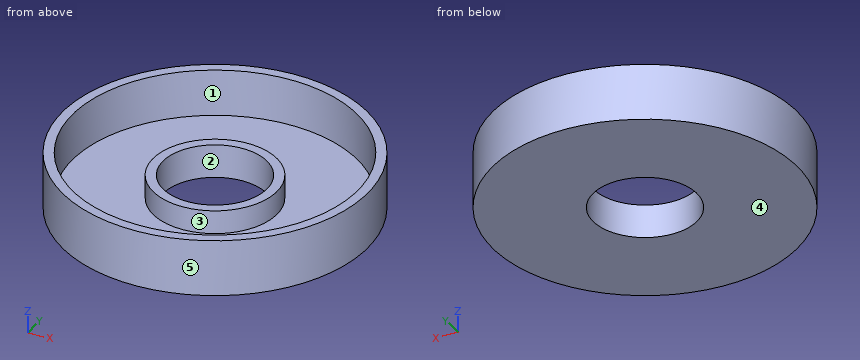
Autodesk Inventor part; units mm, degrees
ref_plane "YZ Plane" through (0, 0, 0) normal (1, 0, 0) x (0, 1, 0)
ref_plane "XZ Plane" through (0, 0, 0) normal (0, 1, 0) x (-1, 0, 0)
ref_plane "XY Plane" through (0, 0, 0) normal (0, 0, 1) x (1, 0, 0)
sketch "Sketch1" plane through (0, 0, 0) normal (0, 0, 1) x (1, 0, 0)
  circle A0 centre (0, 0) radius 61.5
  dimension "d0" = 123
extrude "Extrusion1" add sketch "Sketch1" along normal blind 4
sketch "Sketch2" plane through (0, 0, 4) normal (0, 0, 1) x (1, 0, 0)
  circle A0 centre (0, 0) radius 61.5
  circle A1 centre (0, 0) radius 57.5
  dimension "d12" = 115
extrude "Extrusion2" add sketch "Sketch2" along normal blind 18.85
sketch "Sketch3" plane through (0, 0, 0) normal (0, 0, -1) x (-1, 0, 0)
  circle A0 centre (0, 0) radius 21
  dimension "d6" = 42
extrude "Extrusion3" cut sketch "Sketch3" against normal through all
sketch "Sketch4" plane through (0, 0, 4) normal (0, 0, 1) x (1, 0, 0)
  circle A0 centre (0, 0) radius 21
  circle A1 centre (0, 0) radius 25
  dimension "d9" = 4
extrude "Extrusion4" add sketch "Sketch4" along normal blind 9.5
properties part number "stator_housing"
The listing builds one solid part. Answer for the finished solid, in the listing's coordinates (mm). Face numbers are marked on the shaded views. A direction names the side the tool comes from. Coordinates: 2 decimals unless noted, no trailing zeros. Order: outer loops, then holes, each group sorted by start corner. A loop starts at its lowest first (then second) coordinate and runs counter-clockwise, first axis right, second up.
Q1. Consider line 1 (Y direction, x = 0, z = 6.75); line 2 (Z direction, x = 29, y = -17.5); line 3 (Y direction, x = 0, z = 3.25). Determine where each line is inside the solid, lowest interval first.
Q2. Given P1, Ø15, axis at x = 12, y = -7, coming from the +Z side; P2, Ø12, axis at x = 11.5, z = 13.5, coming from the +Y side; P3, Ø10, axis at x = -47.5, z = 6.5, coming from the -Y side; P4, Ø5, axis at x = 44, y = -33, coming from the -Z side, each flat-ended and moving along its own axis, determine where each tip first touches the part or whether it passes through.
Q3. A cutting plane is placed at C-C, the plane z = 12. Write down the section's boundary in (x, y), and give its area (3 significant figures).
Q4. A cutting plane is placed at A-A, the plane x = 0. Write down the section's boundary in (y, z), and give its area (3 significant figures).
Q5. For a pull along Y with two mould halves and no side action, classify the marked faces 3, 4 and 5 as pulls with the +Y half, pulls with the -Y half, needs draft (parallel to the pull), parting line crosses it, or undercut.
Q6. Which of the six approach directions +Z, -Z, +X, -X, +Y, -Y give full straight-line access (tool end or side, diameter ignored) to the marked faces 1 and 2?
Q7. A cutting plane is placed at D-D, the plane x = 43.5. Write down the section's boundary in (y, z), and give its area (3 significant figures).
Answers follow:
1. line 1: y = -61.5 to -57.5, -25 to -21, 21 to 25, 57.5 to 61.5
1. line 2: z = 0 to 4
1. line 3: y = -61.5 to -21, 21 to 61.5
2. P1: stops at z = 13.5
2. P2: stops at y = 61.25
2. P3: stops at y = -44.45
2. P4: stops at z = 0
3. outline: circle Ø123 at (0, 0); circle Ø50 at (0, 0); hole circle Ø115 at (0, 0); hole circle Ø42 at (0, 0)
3. area: 2,070 mm2
4. outline: (-61.5, 0) - (-21, 0) - (-21, 13.5) - (-25, 13.5) - (-25, 4) - (-57.5, 4) - (-57.5, 22.85) - (-61.5, 22.85) - close; (21, 0) - (61.5, 0) - (61.5, 22.85) - (57.5, 22.85) - (57.5, 4) - (25, 4) - (25, 13.5) - (21, 13.5) - close
4. area: 551 mm2
5. face 3: undercut
5. face 4: needs draft
5. face 5: parting line crosses it
6. face 1: +Z
6. face 2: +Z, -Z
7. outline: (-43.47, 0) - (43.47, 0) - (43.47, 22.85) - (37.6, 22.85) - (37.6, 4) - (-37.6, 4) - (-37.6, 22.85) - (-43.47, 22.85) - close
7. area: 569 mm2
